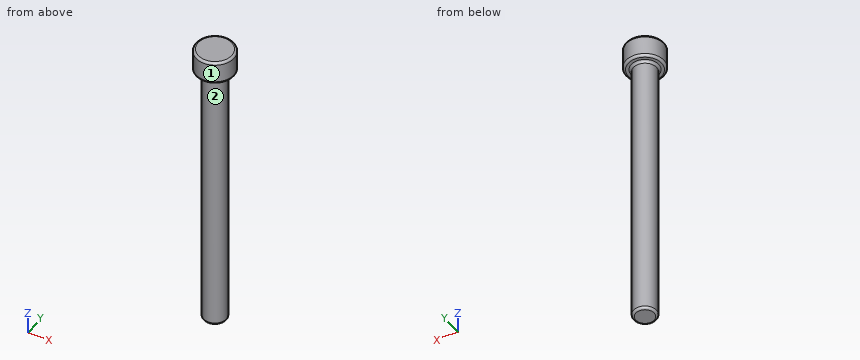
```python
from build123d import *

# Parameters (mm, degrees)
SKETCH1_R           = 2.5
BOSS_EXTRUDE1_DEPTH = 60
SKETCH2_R           = 4.15
BOSS_EXTRUDE2_DEPTH = 5
FILLET1_R           = 0.5


with BuildPart() as part:
    # Sketch1 → Boss-Extrude1 (new body)
    with BuildSketch(Plane.XY):
        Circle(SKETCH1_R)
    extrude(amount=BOSS_EXTRUDE1_DEPTH)

    # Sketch2 → Boss-Extrude2 (add)
    with BuildSketch(Plane.XY.offset(60)):
        Circle(SKETCH2_R)
    extrude(amount=BOSS_EXTRUDE2_DEPTH)

    # Fillet1
    fillet1_edges = [part.edges().sort_by_distance(p)[0] for p in [
        (-2.5, 0, 0),
        (-2.5, 0, 60),
        (-4.15, 0, 60),
        (-4.15, 0, 65),
    ]]
    fillet(fillet1_edges, radius=FILLET1_R)


solid = part.part
```
Here's how the part is built. I have some questions about the finished solid (model axes, mm). Face numbers are marked on the shaded views. A direction names the side the tool comes from. Give positions to 0.01 mm unless a question says otherwise; leave off trailing zeros. Write each loop counter-clockwise with the first axis right and the second up, starting at its lowest first coordinate (ties: lowest second). Pieces come first, ordered by that corner, then holes.
(1) Will these pins go through, and if not, where does the flat tip stop? pin 1 (2 mm diameter, centred on x = 3, z = 41.5, fed in from +Y); pin 2 (2 mm diameter, centred on x = -3, z = 10.5, fed in from -Y); pin 3 (4 mm diameter, centred on y = 1.5, z = 29.5, fed in from -X).
Output values:
pin 1: stops at y = 1.5
pin 2: stops at y = -1.5
pin 3: stops at x = -2.5
(2) On a 3-axis mill with a long thin cutter (end or side, diameter ignored), from which of +Z, -Z, +X, -X, +Y, -Y can I reach the whole of each face in a straight line? I mean the marked faces 1 and 2. Say none if no direction works.
Output values:
face 1: +Z, -Z
face 2: -Z
(3) Imagine slicing it at A-A, the plane y = 0. Write out the boundary of the cut face in (x, z).
Output values:
outline: (-4.15, 60.5) arc R0.5 ccw to (-3.65, 60) - (-3, 60) arc R0.5 cw to (-2.5, 59.5) - (-2.5, 0.5) arc R0.5 ccw to (-2, 0) - (2, 0) arc R0.5 ccw to (2.5, 0.5) - (2.5, 59.5) arc R0.5 cw to (3, 60) - (3.65, 60) arc R0.5 ccw to (4.15, 60.5) - (4.15, 64.5) arc R0.5 ccw to (3.65, 65) - (-3.65, 65) arc R0.5 ccw to (-4.15, 64.5) - close
(4) If I drill on L1, parallel to Z at x = 2.25, y = -3; L2, parallel to X at y = -0.25, z = 12, over which ranges is the centre line in solid material (lowest first)?
Output values:
L1: z = 60.01 to 64.99
L2: x = -2.49 to 2.49
(5) Imagine slicing it at C-C, the plane z = 16. Write out the boundary of the cut face in (x, y), and give its area (3 significant figures).
Output values:
outline: circle Ø5 at (0, 0)
area: 19.6 mm2
